Autodesk Inventor part; units mm, degrees
ref_plane "YZ Plane" through (0, 0, 0) normal (1, 0, 0) x (0, 1, 0)
ref_plane "XZ Plane" through (0, 0, 0) normal (0, 1, 0) x (-1, 0, 0)
ref_plane "XY Plane" through (0, 0, 0) normal (0, 0, 1) x (1, 0, 0)
sketch "Эскиз1" plane through (0, 0, 0) normal (0, 0, 1) x (1, 0, 0)
  circle A0 centre (0, 0) radius 4.5
  circle A1 centre (0, 0) radius 1.75
  line L0 (0, 3.4641) -> (3, 1.7321)
  line L1 (3, 1.7321) -> (3, -1.7321)
  line L2 (3, -1.7321) -> (0, -3.4641)
  line L3 (0, -3.4641) -> (-3, -1.7321)
  line L4 (-3, -1.7321) -> (-3, 1.7321)
  line L5 (-3, 1.7321) -> (0, 3.4641)
  dimension "d0" = 3.5
  dimension "d1" = 9
  dimension "d3" = 6
extrude "Выдавливание1" add sketch "Эскиз1" along normal blind 6 contours A0 | L0 L1 L2 L3 L4 L5
extrude "Выдавливание2" cut sketch "Эскиз1" along normal blind 3.5 contours L0 L1 L2 L3 L4 L5
fillet "Сопряжение1" radius 1 1 edges at (-4.5, 0, 0)
properties part number "Стопор"
Read the model definition and answer for the solid it produces. Units are mm, in the model's axes. A direction names the side the tool comes from. Give positions to 0.01 mm unless a question says otherwise; leave off trailing zeros. Order: outer loops, then holes, each group sorted by start corner. A loop starts at its lowest first (then second) coordinate and runs counter-clockwise, first axis right, second up. Notation, with made-up numbers: (55, 62.25) -> (71, 62.25) arc R8 ccw to (71, 71.25) -> close; hole circle Ø11 at (50.25, 54.25). An arc over 180 degrees is marked (long way). Write item = value, one per line.
1. A cutting plane is placed at C-C, the plane z = 5.15. Write down the section's boundary in (x, y), and give its area (3 significant figures).
Numbers:
outline = circle Ø9 at (0, 0); hole circle Ø3.5 at (0, 0)
area = 54.0 mm²
2. For faces 4 (the face through (1.5, 2.6, 1.7)), 5 (the face through (1.3, 2.9, 0)), determine the directions among +Z, -Z, +X, -X, +Y, -Y from which every point of the face is accessible in a straight line to the end or side of a thin tool.
Numbers:
face_4 = -Z
face_5 = -Z, +X, -X, +Y, -Y
3. A cutting plane is placed at B-B, the plane z = 1.4. Write down the section's boundary in (x, y), and give its area (3 significant figures).
Numbers:
outline = circle Ø9 at (0, 0); hole (-3, -1.73) -> (0, -3.46) -> (3, -1.73) -> (3, 1.73) -> (0, 3.46) -> (-3, 1.73) -> close
area = 32.4 mm²
4. A cutting plane is placed at A-A, the plane y = 0. Write down the section's boundary in (x, z).
Numbers:
outline = (-4.5, 1) arc R1 ccw to (-3.5, 0) -> (-3, 0) -> (-3, 3.5) -> (-1.75, 3.5) -> (-1.75, 6) -> (-4.5, 6) -> close; (1.75, 3.5) -> (3, 3.5) -> (3, 0) -> (3.5, 0) arc R1 ccw to (4.5, 1) -> (4.5, 6) -> (1.75, 6) -> close
5. Straight lines are drawn through the part: line 1 along Y through (x, z) = (0, 4.6); line 2 along X through (y, z) = (-3, 0.8); line 3 along Z through (x, y) = (-2.25, -0.25). For each, find the intervals that lie inside material, in ascending order.
Numbers:
line_1 = -4.5 to -1.75, 1.75 to 4.5
line_2 = -3.33 to -0.8, 0.8 to 3.33
line_3 = 3.5 to 6
6. Given pin 1 (2 mm diameter, centred on y = 3.5, z = 2, fed in from +X); pin 2 (2 mm diameter, centred on x = 3.5, z = 1, fed in from +Y); pin 3 (3 mm diameter, centred on x = 1, y = 0, fed in from -Z), each flat-ended and moving along its own axis, determine where each tip first touches the part or whether it passes through.
Numbers:
pin_1 = 3.74
pin_2 = 3.74
pin_3 = 3.5
7. The mould has two halves that part along Y. Classify faces 1 (the face through (1.5, -2.6, 1.7)), 2 (the face through (0, -2, 6)), 3 (the face through (-0.59, -4.46, 3.46)): +Y half, -Y half, draft (parallel to the pull), parting line (faces both ways), or undercut.
Numbers:
face_1 = undercut
face_2 = draft
face_3 = parting line
